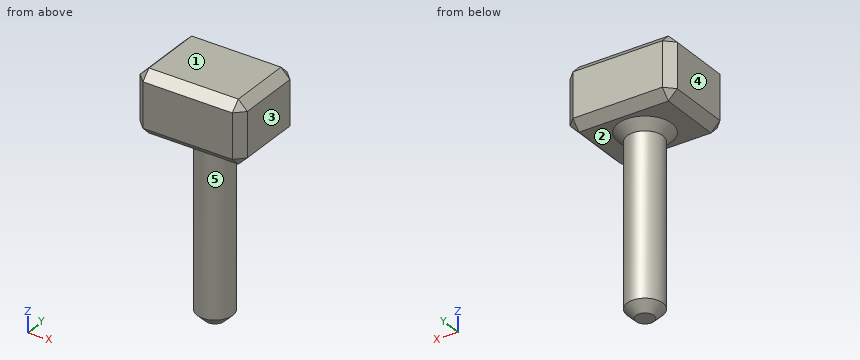
```python
from build123d import *

# Parameters (mm, degrees)
F0_W     = 60
F0_H     = 45
F0_R     = 10
F1_DEPTH = 35
F2_DEPTH = 100
F3_SIZE  = 5
F4_SIZE  = 5


with BuildPart() as f1:
    # F0 (on Top) → F1 (new body)
    with BuildSketch(Plane.XY):
        Rectangle(F0_W, F0_H)
        Circle(F0_R, mode=Mode.SUBTRACT)
        Circle(F0_R)
    extrude(amount=F1_DEPTH)

    # F0 (on Top) → F2 (join)
    with BuildSketch(Plane.XY):
        Circle(F0_R)
    extrude(amount=-F2_DEPTH)

    # F3
    f3_edges = [f1.edges().sort_by_distance(p)[0] for p in [
        (-30, -22.5, 17.5),
        (30, -22.5, 17.5),
        (30, 22.5, 17.5),
        (-30, 22.5, 17.5),
        (0, 22.5, 35),
        (0, 22.5, 0),
        (0, -22.5, 35),
        (0, -22.5, 0),
        (-30, 0, 0),
        (-30, 0, 35),
        (30, 0, 35),
        (30, 0, 0),
    ]]
    chamfer(f3_edges, length=F3_SIZE)

    # F4
    f4_edges = [f1.edges().sort_by_distance(p)[0] for p in [
        (10, 0, -50),
        (-10, 0, 0),
        (-10, 0, -100),
    ]]
    chamfer(f4_edges, length=F4_SIZE)


solid = f1.part
```
Work out the finished part from the listing and answer in its coordinate system (mm). Face numbers are marked on the shaded views. A direction names the side the tool comes from. Round coordinates to 2 decimals unless told otherwise and drop trailing zeros. Write each loop counter-clockwise with the first axis right and the second up, starting at its lowest first coordinate (ties: lowest second). Pieces come first, ordered by that corner, then holes. Notation, with made-up numbers: (-24.75, -27) -> (-18.75, -27) arc R20 ccw to (-18.75, -10) -> close; hole circle Ø7 at (73.5, 32.5). An arc over 180 degrees is marked (long way). Write each question's results on one line, items separated by ' | '.
1) For a pull along Z with two mould halves and no side action, classify the marked faces 1, 2 and 3 as +Z half, -Z half, draft (parallel to the pull), parting line (faces both ways), or undercut.
Findings:
face 1: +Z half | face 2: -Z half | face 3: draft
2) The part is cut by section D-D (x = 21). Write down the section's boundary in (y, z), and give its area (4 significant figures).
Findings:
outline: (-22.5, 5) -> (-17.5, 0) -> (17.5, 0) -> (22.5, 5) -> (22.5, 30) -> (17.5, 35) -> (-17.5, 35) -> (-22.5, 30) -> close | area: 1,525 mm²
3) The part is cut by section B-B (y = 0). Write down the section's boundary in (x, z).
Findings:
outline: (-30, 5) -> (-25, 0) -> (-15, 0) -> (-10, -5) -> (-10, -95) -> (-5, -100) -> (5, -100) -> (10, -95) -> (10, -5) -> (15, 0) -> (25, 0) -> (30, 5) -> (30, 30) -> (25, 35) -> (-25, 35) -> (-30, 30) -> close
4) Which of the six approach directions +Z, -Z, +X, -X, +Y, -Y give full straight-line access (tool end or side, diameter ignored) to the marked faces 4 and 5?
Findings:
face 4: +Z, -Z, -X, +Y, -Y | face 5: -Z
5) Flat-ended cylindrical pins translate along their axes: pin 1 (6 mm diameter, centred on x = 11, z = -11.5, fed in from +Y); pin 2 (10 mm diameter, centred on x = -5.5, y = -12.5, fed in from -Z); pin 3 (3 mm diameter, centred on x = 6, z = -49.5, fed in from +Y). Find the tip coordinate at first contact, or state that the pin passes through.
Findings:
pin 1: stops at y = 6 | pin 2: stops at z = -96.34 | pin 3: stops at y = 8.93
6) Consider line 1 along Z through (x, y) = (12.5, 8.5); line 2 along Y through (x, z) = (-6, -12); line 3 along X through (y, z) = (-3.5, -51.5). Determine where each line is inside the solid, lowest interval first. Write a range as [from, to].
Findings:
line 1: z = [0, 35] | line 2: y = [-8, 8] | line 3: x = [-9.37, 9.37]
7) The part is cut by section C-C (z = -50). Write down the section's boundary in (x, y), and give its area (3 significant figures).
Findings:
outline: circle Ø20 at (0, 0) | area: 314 mm²
8) The part is cut by section A-A (x = 0). Write down the section's boundary in (y, z), and give its area (4 significant figures).
Findings:
outline: (-22.5, 5) -> (-17.5, 0) -> (-15, 0) -> (-10, -5) -> (-10, -95) -> (-5, -100) -> (5, -100) -> (10, -95) -> (10, -5) -> (15, 0) -> (17.5, 0) -> (22.5, 5) -> (22.5, 30) -> (17.5, 35) -> (-17.5, 35) -> (-22.5, 30) -> close | area: 3,525 mm²
